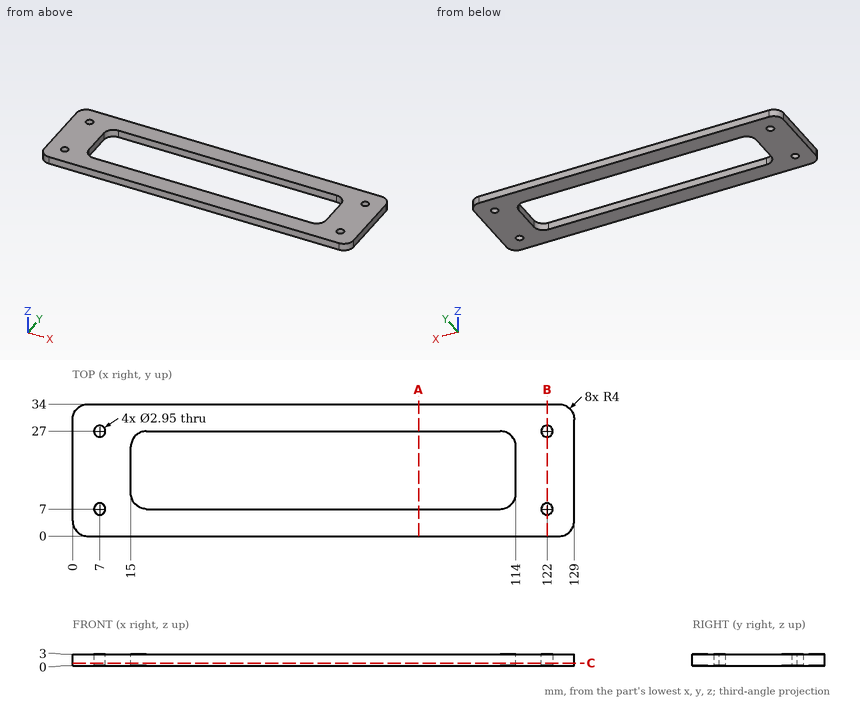
For this review, use the dimensioned drawing (mm, ordinates from the lowest corner) and the shaded views. Round coordinates to 2 decimals unless told otherwise and drop trailing zeros. Write each loop counter-clockwise with the first axis right and the second up, starting at its lowest first coordinate (ties: lowest second). Pieces come first, ordered by that corner, then holes. Notation, with made-up numbers: (13.5, -7) - (63.5, -7) arc R16 cw to (63.5, 22) - close; hole circle Ø9 at (30.5, 46). An arc over 180 degrees is marked (long way). Use a Markdown table: item, result.
Q1. Wall thickness on line 1 along Y through (x, z) = (122, 0.8) (3 decimals); line 2 along Y through (x, z) = (91, 1.95); line 3 along X through (y, z) = (20, 0.35): over which ranges is each line inside the solid? List them lowest first.
Derived:
| item | result |
|---|---|
| line 1 | y = 0 to 5.525, 8.475 to 25.525, 28.475 to 34 |
| line 2 | y = 0 to 7, 27 to 34 |
| line 3 | x = 0 to 15, 114 to 129 |
Q2. Clearance check with flat-ended pins moving along their axes: pin 1 (1.8 mm diameter, centred on x = 7, y = 7, fed in from -Z); pin 2 (4.5 mm diameter, centred on x = 7, y = 27, fed in from -Z). State where each tip first meets the part, or that it passes through.
Derived:
| item | result |
|---|---|
| pin 1 | passes through |
| pin 2 | stops at z = 0 |
Q3. We need section B-B (x = 122). Give the boundary of the cut face in (y, z) (3 decimals).
Derived:
| item | result |
|---|---|
| outline | (0, 0) - (5.525, 0) - (5.525, 3) - (0, 3) - close; (8.475, 0) - (25.525, 0) - (25.525, 3) - (8.475, 3) - close; (28.475, 0) - (34, 0) - (34, 3) - (28.475, 3) - close |
Q4. We need section C-C (z = 0.7). Give the boundary of the cut face in (x, y) (3 decimals).
Derived:
| item | result |
|---|---|
| outline | (0, 4) arc R4 ccw to (4, 0) - (125, 0) arc R4 ccw to (129, 4) - (129, 30) arc R4 ccw to (125, 34) - (4, 34) arc R4 ccw to (0, 30) - close; hole circle Ø2.95 at (7, 7); hole circle Ø2.95 at (7, 27); hole (15, 11) arc R4 ccw to (19, 7) - (110, 7) arc R4 ccw to (114, 11) - (114, 23) arc R4 ccw to (110, 27) - (19, 27) arc R4 ccw to (15, 23) - close; hole circle Ø2.95 at (122, 7); hole circle Ø2.95 at (122, 27) |
Q5. We need section A-A (x = 89). Give the boundary of the cut face in (y, z), plus the area to 3 significant figures.
Derived:
| item | result |
|---|---|
| outline | (0, 0) - (7, 0) - (7, 3) - (0, 3) - close; (27, 0) - (34, 0) - (34, 3) - (27, 3) - close |
| area | 42.0 mm2 |
